```python
from build123d import *

# Parameters (mm, degrees)
BOSS_EXTRUDE1_DEPTH             = 3.175
F_9_64_0_14063_DIAMETER_HOLE1_D = 3.572002
F_9_64_0_14063_DIAMETER_HOLE2_D = 3.572002


with BuildPart() as part:
    # Sketch1 → Boss-Extrude1 (new body)
    with BuildSketch(Plane.XY):
        with BuildLine():
            Line((0, -4.7625), (-76.2, -4.7625))
            ThreePointArc((-76.2, -4.7625), (-80.9625, 0), (-76.2, 4.7625))
            Line((-76.2, 4.7625), (0, 4.7625))
            ThreePointArc((0, 4.7625), (4.7625, 0), (0, -4.7625))
        make_face()
    extrude(amount=BOSS_EXTRUDE1_DEPTH)

    # 9/64 (0.14063) Diameter Hole1 (through all)
    with Locations(Plane.XY.offset(3.175)):
        with Locations((0, 0), (-76.2, 0)):
            Hole(F_9_64_0_14063_DIAMETER_HOLE1_D / 2)

    # 9/64 (0.14063) Diameter Hole2 (through all)
    with Locations(Plane.XY.offset(3.175)):
        with Locations((-12.7, 0), (-63.5, 0)):
            Hole(F_9_64_0_14063_DIAMETER_HOLE2_D / 2)


solid = part.part
```
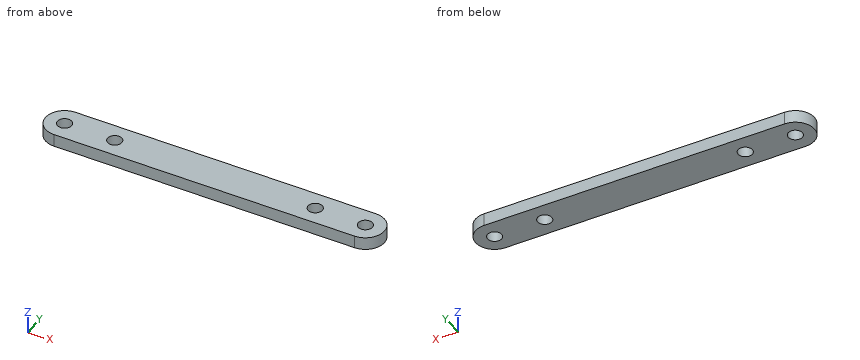
The listing builds one solid part. Answer for the finished solid, in the listing's coordinates (mm). Round coordinates to 2 decimals unless told otherwise and drop trailing zeros. Loops run counter-clockwise (first coordinate to the right, second up) from the corner with the lowest first, then second, coordinate; pieces in that order, holes last.
Q1. Section D-D, the plane x = -12 is taken. Determine the outline of the cut face in (y, z) (1 decimal), then the cut area to 3 significant figures.
Q2. Section A-A, the plane y = 0 is taken. Determine the outline of the cut face in (x, z) (1 decimal).
Q3. Section B-B, the plane x = -63.5 is taken. Determine the outline of the cut face in (y, z) (1 decimal), then the cut area to 3 significant figures.
Q4. Given pin 1 Ø2 at (x, y) = (0, 0) entering from -Z, flat-ended and moving along its own axis, determine where the tip first touches the part or whether it passes through.
Q5. Section C-C, the plane z = 1.05 is taken. Determine the outline of the cut face in (x, y) (1 decimal).
Q6. Find the intervals of material crossed by line 1 (X direction, y = -0.25, z = 0.3); line 2 (Y direction, x = -76.2, z = 1.35); line 3 (X direction, y = 0.5, z = 0.6), in increasing order.
Completed:
1. outline: (-4.8, 0) - (-1.6, 0) - (-1.6, 3.2) - (-4.8, 3.2) - close; (1.6, 0) - (4.8, 0) - (4.8, 3.2) - (1.6, 3.2) - close
1. area: 19.8 mm2
2. outline: (-81, 0) - (-78, 0) - (-78, 3.2) - (-81, 3.2) - close; (-74.4, 0) - (-65.3, 0) - (-65.3, 3.2) - (-74.4, 3.2) - close; (-61.7, 0) - (-14.5, 0) - (-14.5, 3.2) - (-61.7, 3.2) - close; (-10.9, 0) - (-1.8, 0) - (-1.8, 3.2) - (-10.9, 3.2) - close; (1.8, 0) - (4.8, 0) - (4.8, 3.2) - (1.8, 3.2) - close
3. outline: (-4.8, 0) - (-1.8, 0) - (-1.8, 3.2) - (-4.8, 3.2) - close; (1.8, 0) - (4.8, 0) - (4.8, 3.2) - (1.8, 3.2) - close
3. area: 18.9 mm2
4. pin 1: passes through
5. outline: (-76.2, -4.8) - (0, -4.8) arc R4.8 ccw to (0, 4.8) - (-76.2, 4.8) arc R4.8 ccw to start; hole circle Ø3.6 at (-76.2, 0); hole circle Ø3.6 at (-63.5, 0); hole circle Ø3.6 at (-12.7, 0); hole circle Ø3.6 at (0, 0)
6. line 1: x = -80.96 to -77.97, -74.43 to -65.27, -61.73 to -14.47, -10.93 to -1.77, 1.77 to 4.76
6. line 2: y = -4.76 to -1.79, 1.79 to 4.76
6. line 3: x = -80.94 to -77.91, -74.49 to -65.21, -61.79 to -14.41, -10.99 to -1.71, 1.71 to 4.74
